Build history of the part. All positions in model axes, mm. A direction names the side the tool comes from. Round coordinates to 2 decimals unless told otherwise and drop trailing zeros. Order: outer loops, then holes, each group sorted by start corner. A loop starts at its lowest first (then second) coordinate and runs counter-clockwise, first axis right, second up. Notation, with made-up numbers: (11, 47) -> (59, 47) arc R30 cw to (59, 81) -> close; hole circle Ø11 at (-10, 78.25). An arc over 180 degrees is marked (long way). Use a Markdown table: item, result. Add a question column.
Item 1: Pin check, flat tips, straight feed: pin 1 (1.5 mm diameter, centred on y = 3.5, z = 5, fed in from -X); pin 2 (4 mm diameter, centred on x = 0.5, z = 5, fed in from +Y); pin 3 (1.2 mm diameter, centred on x = 0.5, y = 5, fed in from +Z); pin 4 (0.7 mm diameter, centred on x = 0.5, y = 7, fed in from +Z). Stop position of each tip, or through.
Item 2: 3-axis set-ups, long thin cutter, end or side, ignore diameter. For faces 5 (the face through (0.7, 5.3, -1.5)), 6 (the face through (1, 7, 1.95)), 7 (the face through (1.78, 1.09, -0.11)): which of +Z, -Z, +X, -X, +Y, -Y reach the whole face in a straight line?
Item 3: Slice it at A-A, the plane z = -0.5. Give the cut face in (x, y).
Item 4: Probe L1, parallel to X at y = 2.5, z = 6.25; L2, parallel to X at y = 0.5, z = -4.75; L3, parallel to Y at x = -5.25, z = -4.5. List the from-to ranges inside material, lowest first.
Item 5: Two-plate mould, pull along X, no slides. Class faces 1 (the face through (0.82, 6.01, -1.78)), 2 (the face through (-7.055, 2.921, -7.443)), 3 (the face through (2.84, 6.64, -0.03)), 4 (the face through (0, 2.8, 0)): released by +X, released by -X, zero draft, split by the parting line, or undercut.
Item 6: Slice it at B-B, the plane z = -5.25. Give the cut face in (x, y), plus the area to 3 significant figures.
from build123d import *

# Parameters (mm, degrees)
EXTRUDE_1_DEPTH      = 7.5
EXTRUDE_1_DEPTH_BACK = 7.5
EXTRUDE_2_DEPTH      = 1.5
EXTRUDE_2_DEPTH_BACK = 1.5
EXTRUDE_3_DEPTH      = 2
EXTRUDE_3_DEPTH_BACK = 2
CUT_EXTRUDE_1_DEPTH  = 15.42315829
FILLET_1_R           = 0.2
FILLET_2_R           = 0.1


with BuildPart() as part:
    # 草图1 → 凸台-拉伸1 (new, two sides: drawn at the far end of the back side and taken through both)
    with BuildSketch(Plane.XY.offset(-EXTRUDE_1_DEPTH_BACK)):
        with BuildLine():
            Line((-7.5, 0), (-1.5, 0))
            Line((-1.5, 0), (-1.5, 0.677124344))
            ThreePointArc((-1.5, 0.677124344), (-1.780042303, 1.088161527), (-1.95, 1.555590279))
            Line((-1.95, 1.555590279), (-1.95, 2.8))
            Line((-1.95, 2.8), (1.95, 2.8))
            Line((1.95, 2.8), (1.95, 1.555590279))
            ThreePointArc((1.95, 1.555590279), (1.780042303, 1.088161527), (1.5, 0.677124344))
            Line((1.5, 0.677124344), (1.5, 0))
            Line((1.5, 0), (7.5, 0))
            Line((7.5, 0), (8.022104769, 3.965779445))
            Line((8.022104769, 3.965779445), (-6.722338928, 5.906922284))
            Line((-6.722338928, 5.906922284), (-7.5, 0))
        make_face()
    extrude(amount=EXTRUDE_1_DEPTH + EXTRUDE_1_DEPTH_BACK)

    # 草图2 → 凸台-拉伸2 (add, two sides: drawn at the far end of the back side and taken through both)
    with BuildSketch(Plane.XY.offset(-EXTRUDE_2_DEPTH_BACK)):
        Polygon((-0.837284372, 5.132140153), (2.137050212, 4.740561576), (2.267576405, 5.732006438), (-0.70675818, 6.123585014), align=None)
    extrude(amount=EXTRUDE_2_DEPTH + EXTRUDE_2_DEPTH_BACK)

    # 草图3 → 凸台-拉伸3 (add, two sides: drawn at the far end of the back side and taken through both)
    with BuildSketch(Plane.XY.offset(-EXTRUDE_3_DEPTH_BACK)):
        with BuildLine():
            Line((-0.957119079, 7.669489093), (-1.080389284, 6.733158928))
            ThreePointArc((-1.080389284, 6.733158928), (-0.972897293, 6.247545163), (-0.748901909, 5.803471605))
            Line((-0.748901909, 5.803471605), (2.225432675, 5.411893028))
            ThreePointArc((2.225432675, 5.411893028), (2.556730295, 5.782860875), (2.786245676, 6.224106778))
            Line((2.786245676, 6.224106778), (2.909515881, 7.160436943))
            Line((2.909515881, 7.160436943), (-0.957119079, 7.669489093))
        make_face()
    extrude(amount=EXTRUDE_3_DEPTH + EXTRUDE_3_DEPTH_BACK)

    # 草图4 → 切除-拉伸1 (cut, through all)
    with BuildSketch(Plane(origin=(1.93331748, -0.254526075, 0), x_dir=(0, 0, -1), z_dir=(0.9914448613738126, -0.13052619222003545, 0))):
        with BuildLine():
            Line((1.95, 7.478946442), (2, 7.478946442))
            Line((2, 7.478946442), (2, 5.656070786))
            Line((2, 5.656070786), (1.5, 5.656070786))
            ThreePointArc((1.5, 5.656070786), (1.780042303, 6.067107969), (1.95, 6.534536721))
            Line((1.95, 6.534536721), (1.95, 7.478946442))
        make_face()
        with BuildLine():
            Line((-1.95, 7.478946442), (-1.95, 6.534536721))
            ThreePointArc((-1.95, 6.534536721), (-1.780042303, 6.067107969), (-1.5, 5.656070786))
            Line((-1.5, 5.656070786), (-2, 5.656070786))
            Line((-2, 5.656070786), (-2, 7.478946442))
            Line((-2, 7.478946442), (-1.95, 7.478946442))
        make_face()
    extrude(amount=-CUT_EXTRUDE_1_DEPTH, mode=Mode.SUBTRACT)

    # 圆角1
    fillet_1_edges = [part.edges().sort_by_distance(p)[0] for p in [
        (-6.722338928, 5.906922284, 0),
        (8.022104769, 3.965779445, 0),
        (7.5, 0, 0),
        (1.5, 0, 0),
        (-1.5, 0, 0),
        (-7.5, 0, 0),
        (4.5, 0, -7.5),
        (-7.111169464, 2.953461142, 7.5),
        (-4.5, 0, 7.5),
        (7.761052384, 1.982889723, -7.5),
        (4.5, 0, 7.5),
        (7.761052384, 1.982889723, 7.5),
        (0.64988292, 4.936350865, 7.5),
        (0.64988292, 4.936350865, -7.5),
        (-7.111169464, 2.953461142, -7.5),
        (-4.5, 0, -7.5),
    ]]
    fillet(fillet_1_edges, radius=FILLET_1_R)

    # 圆角2
    fillet_2_edges = [part.edges().sort_by_distance(p)[0] for p in [
        (2.909515881, 7.160436943, 0),
        (-0.957119079, 7.669489093, 0),
        (0.976198401, 7.414963018, -1.95),
        (0.976198401, 7.414963018, 1.95),
    ]]
    fillet(fillet_2_edges, radius=FILLET_2_R)


solid = part.part
Check sheet entries:
| question | item | result |
|---|---|---|
| 1 | pin 1 | x = -7.14 |
| 1 | pin 2 | y = 5.22 |
| 1 | pin 3 | z = 7.5 |
| 1 | pin 4 | z = 1.95 |
| 2 | face 5 | -Z |
| 2 | face 6 | +Z, +X, -X, +Y |
| 2 | face 7 | +Z, -Z |
| 3 | outline | (-7.47, 0.23) arc R0.2 ccw to (-7.27, 0) -> (-1.7, 0) arc R0.2 ccw to (-1.5, 0.2) -> (-1.5, 0.68) arc R2 cw to (-1.95, 1.56) -> (-1.95, 2.8) -> (1.95, 2.8) -> (1.95, 1.56) arc R2 cw to (1.5, 0.68) -> (1.5, 0.2) arc R0.2 ccw to (1.7, 0) -> (7.32, 0) arc R0.2 ccw to (7.52, 0.17) -> (8, 3.77) arc R0.2 ccw to (7.82, 3.99) -> (2.14, 4.74) -> (2.23, 5.41) arc R2 ccw to (2.79, 6.22) -> (2.9, 7.06) arc R0.1 ccw to (2.81, 7.17) -> (-0.86, 7.66) arc R0.1 ccw to (-0.97, 7.57) -> (-1.08, 6.73) arc R2 ccw to (-0.75, 5.8) -> (-0.84, 5.13) -> (-6.52, 5.88) arc R0.2 ccw to (-6.75, 5.71) -> close |
| 4 | L1 | -7.17 to -1.95, 1.95 to 7.83 |
| 4 | L2 | -7.43 to -1.5, 1.5 to 7.57 |
| 4 | L3 | 0 to 5.71 |
| 5 | face 1 | undercut |
| 5 | face 2 | released by -X |
| 5 | face 3 | released by +X |
| 5 | face 4 | undercut |
| 6 | outline | (-7.47, 0.23) arc R0.2 ccw to (-7.27, 0) -> (-1.7, 0) arc R0.2 ccw to (-1.5, 0.2) -> (-1.5, 0.68) arc R2 cw to (-1.95, 1.56) -> (-1.95, 2.8) -> (1.95, 2.8) -> (1.95, 1.56) arc R2 cw to (1.5, 0.68) -> (1.5, 0.2) arc R0.2 ccw to (1.7, 0) -> (7.32, 0) arc R0.2 ccw to (7.52, 0.17) -> (8, 3.77) arc R0.2 ccw to (7.82, 3.99) -> (-6.52, 5.88) arc R0.2 ccw to (-6.75, 5.71) -> close |
| 6 | area | 64.0 mm2 |
